Design review of the part built by this model. Coordinates are the model's own, in mm. A direction names the side the tool comes from. Coordinates: 2 decimals unless noted, no trailing zeros. Loops run counter-clockwise (first coordinate to the right, second up) from the corner with the lowest first, then second, coordinate; pieces in that order, holes last. Notation, with made-up numbers: (36.25, -27.75) - (55.25, -27.75) arc R25 ccw to (55.25, -2.75) - close; hole circle Ø7 at (29, -1). An arc over 180 degrees is marked (long way). Answer in a Markdown table with one row per item. Add a question column.
(1) For faces 4 (the face through (11.2, 1, 1.1)), 5 (the face through (9, -4.8, 15)), 6 (the face through (9.954, -11.879, 1.085)), 7 (the face through (10.301, 0, 17)), 8 (the face through (9, 4.8, 26)), list the 3-axis set-ups (+Z, -Z, +X, -X, +Y, -Y) from which the entire face can be reached by the end or side of a thin tool; tool diameter is ignored.
(2) We need section B-B, the plane z = 17. Write out the cut boundary in (x, y), plus the area to 3 significant figures.
(3) We need section D-D, the plane z = 10.25. Write out the cut boundary in (x, y).
(4) The part is to be moulded in two halves that separate along Y. For faces 1 (the face through (9, 3, 24.5)), 2 (the face through (15, 0, 0)), 3 (the face through (3, 21.056, 2)), say which applies: released by +Y, released by -Y, zero draft, split by the parting line, or undercut.
(5) We need section C-C, the plane y = 3.5. Write out the cut boundary in (x, z), plus the area to 3 significant figures.
(6) We need section A-A, the plane x = 0. Write out the cut boundary in (y, z), plus the area to 3 significant figures.
(7) Clearance check with flat-ended pins moving along their axes: pin 1 (5 mm diameter, centred on x = 0, y = 0, fed in from +Z); pin 2 (1.9 mm diameter, centred on x = 9.5, y = 3.5, fed in from +Z); pin 3 (2.5 mm diameter, centred on x = 9, z = 20.5, fed in from -Y); pin 4 (8 mm diameter, centred on x = 10.5, z = 6, fed in from -Y). State where each tip first meets the part, or that it passes through.
(8) To check wall thickness, follow L1, parallel to Y at x = 0, z = 2.9; L2, parallel to Y at x = 0, z = 4.6; L3, parallel to X at y = 0, z = 3.7. State the ranges of each line that lie inside material, in increasing order. Write a range as [from, to].
from build123d import *

# Parameters (mm, degrees)
BOSS_EXTRUDE1_DEPTH   = 2.2
BOSS_EXTRUDE1_2_DEPTH = 2.2
BOSS_EXTRUDE1_3_DEPTH = 2.2
SKETCH3_R             = 1.5
BOSS_EXTRUDE2_DEPTH   = 2.5
SKETCH4_R             = 3.05
CUT_EXTRUDE1_DEPTH    = 0.6
SKETCH5_W             = 2.4
SKETCH5_H             = 2.4
BOSS_EXTRUDE3_DEPTH   = 22.15
BOSS_EXTRUDE4_DEPTH   = 2.4
CHAMFER1_SIZE         = 2
CHAMFER1_SIZE_2       = 1.48467926


with BuildPart() as part:
    # Sketch1 → Boss-Extrude1 (new body)
    with BuildSketch(Plane.XY):
        Polygon((-3.5, 21.055685406), (-3.5, 10.2), (5.888972746, 10.2), (6.342667922, 9.414176903), (13.466375906, 14.276390289), (8.839237969, 21.055685406), align=None)
    extrude(amount=BOSS_EXTRUDE1_DEPTH)



with BuildPart() as body_2:
    # Sketch1 → Boss-Extrude1 2 (new body)
    with BuildSketch(Plane.XY):
        Polygon((18.201821848, -7.338411352), (10.554607275, -2.118883945), (11.777945491, 0), (10.554607275, 2.118883945), (18.201821848, 7.338411352), align=None)
    extrude(amount=BOSS_EXTRUDE1_2_DEPTH)


with BuildPart() as body_3:
    # Sketch1 → Boss-Extrude1 3 (new body)
    with BuildSketch(Plane.XY):
        Polygon((8.839237969, -21.055685406), (13.466375906, -14.276390289), (6.342667922, -9.414176903), (5.888972746, -10.2), (-3.5, -10.2), (-3.5, -21.055685406), align=None)
    extrude(amount=BOSS_EXTRUDE1_3_DEPTH)


with BuildPart() as part_1:
    add(part.part)

    add(body_2.part)  # Boss-Extrude2 merges body 2

    add(body_3.part)  # Boss-Extrude2 merges body 3
    # Sketch3 → Boss-Extrude2 (add)
    with BuildSketch(Plane.XY.offset(2.2)):
        Polygon((-3.5, 21.055685406), (-3.5, -21.055685406), (8.839237969, -21.055685406), (18.201821848, -7.338411352), (18.201821848, 7.338411352), (8.839237969, 21.055685406), align=None)
        Circle(SKETCH3_R, mode=Mode.SUBTRACT)
    extrude(amount=BOSS_EXTRUDE2_DEPTH)

    # Sketch4 → Cut-Extrude1 (cut)
    with BuildSketch(Plane.XY.offset(4.7)):
        Circle(SKETCH4_R)
    extrude(amount=-CUT_EXTRUDE1_DEPTH, mode=Mode.SUBTRACT)

    # Sketch5 → Boss-Extrude3 (add)
    with BuildSketch(Plane.XY.offset(4.7)):
        with Locations((9.100910924, 6)):
            Rectangle(SKETCH5_W, SKETCH5_H)
        with Locations((9.100910924, -6)):
            Rectangle(SKETCH5_W, SKETCH5_H)
    extrude(amount=BOSS_EXTRUDE3_DEPTH)

    # Sketch6 → Boss-Extrude4 (add)
    with BuildSketch(Plane(origin=(10.300910924, 0, 0), x_dir=(0, 0, -1), z_dir=(1, 0, 0))):
        Polygon((-6.387662753, 4.8), (-9.65, -1.526957086), (-12.912337247, 4.8), (-16.287662753, 4.8), (-19.55, -1.526957086), (-22.812337247, 4.8), (-24.5, 4.8), (-24.5, 1.526957086), (-21.237662753, -4.8), (-17.862337247, -4.8), (-14.6, 1.526957086), (-11.337662753, -4.8), (-7.962337247, -4.8), (-4.7, 1.526957086), (-4.7, 4.8), align=None)
    extrude(amount=-BOSS_EXTRUDE4_DEPTH)

    # Chamfer1
    # the kernel refuses this chamfer: 2, 1.48467926 mm, written as the material it adds along each edge
    with BuildSketch(Plane(origin=(15.4442769, 1.526957086, 4.7), x_dir=(0, -1, 0), z_dir=(-1, 0, 0))) as chamfer1_piece_1_section:
        Polygon((CHAMFER1_SIZE, 0), (CHAMFER1_SIZE_2 * 0.888803167403, CHAMFER1_SIZE_2 * 0.458289133192), (0, 0), align=None)
    chamfer1_piece_1 = extrude(amount=12.686731952, mode=Mode.PRIVATE)
    chamfer1_piece_1 = split(chamfer1_piece_1, bisect_by=Plane(origin=(10.672593912, 1.526957086, 9.471682988), z_dir=(0.7071067811865476, 0, -0.7071067811865476)), keep=Keep.TOP, mode=Mode.PRIVATE)
    chamfer1_piece_1 = split(chamfer1_piece_1, bisect_by=Plane(origin=(13.872593912, 1.526957086, 3.128317012), z_dir=(-0.7071067811865476, 0, -0.7071067811865476)), keep=Keep.TOP, mode=Mode.PRIVATE)
    add(chamfer1_piece_1)
    with BuildSketch(Plane(origin=(2.757544948, 7.2, 4.7), x_dir=(0, 1, 0), z_dir=(1, 0, 0))) as chamfer1_piece_2_section:
        Polygon((CHAMFER1_SIZE, 0), (0, CHAMFER1_SIZE), (0, 0), align=None)
    chamfer1_piece_2 = extrude(amount=12.686731952, mode=Mode.PRIVATE)
    chamfer1_piece_2 = split(chamfer1_piece_2, bisect_by=Plane(origin=(4.329227936, 7.2, 3.128317012), z_dir=(0.7071067811865476, 0, -0.7071067811865476)), keep=Keep.TOP, mode=Mode.PRIVATE)
    chamfer1_piece_2 = split(chamfer1_piece_2, bisect_by=Plane(origin=(7.529227936, 7.2, 9.471682988), z_dir=(-0.7071067811865476, 0, -0.7071067811865476)), keep=Keep.TOP, mode=Mode.PRIVATE)
    add(chamfer1_piece_2)
    with BuildSketch(Plane(origin=(10.300910924, 12.343365976, 4.7), x_dir=(1, 0, 0), z_dir=(0, -1, 0))) as chamfer1_piece_3_section:
        Polygon((CHAMFER1_SIZE, 0), (0, CHAMFER1_SIZE), (0, 0), align=None)
    chamfer1_piece_3 = extrude(amount=15.959774866, mode=Mode.PRIVATE)
    chamfer1_piece_3 = split(chamfer1_piece_3, bisect_by=Plane(origin=(10.300910924, 4.8, 4.7), z_dir=(0, 1, 0)), keep=Keep.TOP, mode=Mode.PRIVATE)
    chamfer1_piece_3 = split(chamfer1_piece_3, bisect_by=Plane(origin=(10.300910924, 10.771682988, 3.128317012), z_dir=(0, -0.7071067811865476, -0.7071067811865476)), keep=Keep.TOP, mode=Mode.PRIVATE)
    add(chamfer1_piece_3)
    with BuildSketch(Plane(origin=(10.300910924, 12.343365976, 4.7), x_dir=(1, 0, 0), z_dir=(0, -1, 0))) as chamfer1_piece_4_section:
        Polygon((CHAMFER1_SIZE, 0), (0, CHAMFER1_SIZE), (0, 0), align=None)
    chamfer1_piece_4 = extrude(amount=15.959774866, mode=Mode.PRIVATE)
    chamfer1_piece_4 = split(chamfer1_piece_4, bisect_by=Plane(origin=(10.300910924, 11.446474594, 2.96057429), z_dir=(0, -0.4582891331950048, -0.8888031674084939)), keep=Keep.TOP, mode=Mode.PRIVATE)
    chamfer1_piece_4 = split(chamfer1_piece_4, bisect_by=Plane(origin=(10.300910924, 5.935161531, 11.108204445), z_dir=(0, 0.7071067811865488, -0.7071067811865462)), keep=Keep.TOP, mode=Mode.PRIVATE)
    add(chamfer1_piece_4)
    with BuildSketch(Plane(origin=(10.300910924, 12.343365976, 4.7), x_dir=(1, 0, 0), z_dir=(0, -1, 0))) as chamfer1_piece_5_section:
        Polygon((CHAMFER1_SIZE, 0), (0, CHAMFER1_SIZE), (0, 0), align=None)
    chamfer1_piece_5 = extrude(amount=15.959774866, mode=Mode.PRIVATE)
    chamfer1_piece_5 = split(chamfer1_piece_5, bisect_by=Plane(origin=(10.300910924, 10.071607195, 0.294164788), z_dir=(0, 0.4582891331950048, 0.8888031674084939)), keep=Keep.TOP, mode=Mode.PRIVATE)
    chamfer1_piece_5 = split(chamfer1_piece_5, bisect_by=Plane(origin=(10.300910924, 5.935161531, 11.108204445), z_dir=(0, -0.7071067811865488, 0.7071067811865462)), keep=Keep.TOP, mode=Mode.PRIVATE)
    add(chamfer1_piece_5)
    with BuildSketch(Plane(origin=(7.900910924, -3.61640889, 4.7), x_dir=(-1, 0, 0), z_dir=(0, 1, 0))) as chamfer1_piece_6_section:
        Polygon((CHAMFER1_SIZE, 0), (0, CHAMFER1_SIZE), (0, 0), align=None)
    chamfer1_piece_6 = extrude(amount=15.959774866, mode=Mode.PRIVATE)
    chamfer1_piece_6 = split(chamfer1_piece_6, bisect_by=Plane(origin=(7.900910924, -2.53615324, 6.795041262), z_dir=(0, 0.4582891331950048, 0.8888031674084939)), keep=Keep.TOP, mode=Mode.PRIVATE)
    chamfer1_piece_6 = split(chamfer1_piece_6, bisect_by=Plane(origin=(7.900910924, -1.16128584, 9.461450764), z_dir=(0, -0.4582891331950048, -0.8888031674084939)), keep=Keep.TOP, mode=Mode.PRIVATE)
    add(chamfer1_piece_6)
    with BuildSketch(Plane(origin=(7.900910924, -3.61640889, 4.7), x_dir=(-1, 0, 0), z_dir=(0, 1, 0))) as chamfer1_piece_7_section:
        Polygon((CHAMFER1_SIZE, 0), (0, CHAMFER1_SIZE), (0, 0), align=None)
    chamfer1_piece_7 = extrude(amount=15.959774866, mode=Mode.PRIVATE)
    chamfer1_piece_7 = split(chamfer1_piece_7, bisect_by=Plane(origin=(7.900910924, -1.16128584, 9.461450764), z_dir=(0, -0.4582891331950048, -0.8888031674084939)), keep=Keep.TOP, mode=Mode.PRIVATE)
    chamfer1_piece_7 = split(chamfer1_piece_7, bisect_by=Plane(origin=(7.900910924, -2.044725902, 3.128317012), z_dir=(0, 0.7071067811865488, -0.7071067811865462)), keep=Keep.TOP, mode=Mode.PRIVATE)
    add(chamfer1_piece_7)
    with BuildSketch(Plane(origin=(7.900910924, -3.61640889, 4.7), x_dir=(-1, 0, 0), z_dir=(0, 1, 0))) as chamfer1_piece_8_section:
        Polygon((CHAMFER1_SIZE, 0), (0, CHAMFER1_SIZE), (0, 0), align=None)
    chamfer1_piece_8 = extrude(amount=15.959774866, mode=Mode.PRIVATE)
    chamfer1_piece_8 = split(chamfer1_piece_8, bisect_by=Plane(origin=(7.900910924, 4.8, 4.7), z_dir=(0, 1, 0)), keep=Keep.TOP, mode=Mode.PRIVATE)
    chamfer1_piece_8 = split(chamfer1_piece_8, bisect_by=Plane(origin=(7.900910924, 2.791795555, 11.108204445), z_dir=(0, -0.7071067811865476, -0.7071067811865476)), keep=Keep.TOP, mode=Mode.PRIVATE)
    add(chamfer1_piece_8)
    with BuildSketch(Plane(origin=(2.757544948, -4.8, 4.7), x_dir=(0, 1, 0), z_dir=(1, 0, 0))) as chamfer1_piece_9_section:
        Polygon((CHAMFER1_SIZE, 0), (0, CHAMFER1_SIZE), (0, 0), align=None)
    chamfer1_piece_9 = extrude(amount=12.686731952, mode=Mode.PRIVATE)
    chamfer1_piece_9 = split(chamfer1_piece_9, bisect_by=Plane(origin=(4.329227936, -4.8, 3.128317012), z_dir=(0.7071067811865476, 0, -0.7071067811865476)), keep=Keep.TOP, mode=Mode.PRIVATE)
    chamfer1_piece_9 = split(chamfer1_piece_9, bisect_by=Plane(origin=(7.529227936, -4.8, 9.471682988), z_dir=(-0.7071067811865476, 0, -0.7071067811865476)), keep=Keep.TOP, mode=Mode.PRIVATE)
    add(chamfer1_piece_9)
    with BuildSketch(Plane(origin=(10.300910924, 0.343365976, 4.7), x_dir=(1, 0, 0), z_dir=(0, -1, 0))) as chamfer1_piece_10_section:
        Polygon((CHAMFER1_SIZE, 0), (0, CHAMFER1_SIZE), (0, 0), align=None)
    chamfer1_piece_10 = extrude(amount=12.686731952, mode=Mode.PRIVATE)
    chamfer1_piece_10 = split(chamfer1_piece_10, bisect_by=Plane(origin=(10.300910924, 0.59195435, 5.182110786), z_dir=(0, 0.4582891331950048, 0.8888031674084939)), keep=Keep.TOP, mode=Mode.PRIVATE)
    add(chamfer1_piece_10)
    with BuildSketch(Plane(origin=(10.300910924, 0.343365976, 4.7), x_dir=(1, 0, 0), z_dir=(0, -1, 0))) as chamfer1_piece_11_section:
        Polygon((CHAMFER1_SIZE, 0), (0, CHAMFER1_SIZE), (0, 0), align=None)
    chamfer1_piece_11 = extrude(amount=12.686731952, mode=Mode.PRIVATE)
    chamfer1_piece_11 = split(chamfer1_piece_11, bisect_by=Plane(origin=(10.300910924, -4.428317012, 9.471682988), z_dir=(0, 0.7071067811865477, -0.7071067811865474)), keep=Keep.TOP, mode=Mode.PRIVATE)
    chamfer1_piece_11 = split(chamfer1_piece_11, bisect_by=Plane(origin=(10.300910924, -1.228317012, 3.128317012), z_dir=(0, -0.7071067811865476, -0.7071067811865476)), keep=Keep.TOP, mode=Mode.PRIVATE)
    add(chamfer1_piece_11)
    with BuildSketch(Plane(origin=(15.4442769, -7.2, 4.7), x_dir=(0, -1, 0), z_dir=(-1, 0, 0))) as chamfer1_piece_12_section:
        Polygon((CHAMFER1_SIZE, 0), (0, CHAMFER1_SIZE), (0, 0), align=None)
    chamfer1_piece_12 = extrude(amount=12.686731952, mode=Mode.PRIVATE)
    chamfer1_piece_12 = split(chamfer1_piece_12, bisect_by=Plane(origin=(10.672593912, -7.2, 9.471682988), z_dir=(0.7071067811865476, 0, -0.7071067811865476)), keep=Keep.TOP, mode=Mode.PRIVATE)
    chamfer1_piece_12 = split(chamfer1_piece_12, bisect_by=Plane(origin=(13.872593912, -7.2, 3.128317012), z_dir=(-0.7071067811865476, 0, -0.7071067811865476)), keep=Keep.TOP, mode=Mode.PRIVATE)
    add(chamfer1_piece_12)
    with BuildSketch(Plane(origin=(7.900910924, -12.343365976, 4.7), x_dir=(-1, 0, 0), z_dir=(0, 1, 0))) as chamfer1_piece_13_section:
        Polygon((CHAMFER1_SIZE, 0), (0, CHAMFER1_SIZE), (0, 0), align=None)
    chamfer1_piece_13 = extrude(amount=12.686731952, mode=Mode.PRIVATE)
    chamfer1_piece_13 = split(chamfer1_piece_13, bisect_by=Plane(origin=(7.900910924, -10.771682988, 3.128317012), z_dir=(0, 0.7071067811865477, -0.7071067811865474)), keep=Keep.TOP, mode=Mode.PRIVATE)
    chamfer1_piece_13 = split(chamfer1_piece_13, bisect_by=Plane(origin=(7.900910924, -7.571682988, 9.471682988), z_dir=(0, -0.7071067811865476, -0.7071067811865476)), keep=Keep.TOP, mode=Mode.PRIVATE)
    add(chamfer1_piece_13)
    with BuildSketch(Plane(origin=(7.900910924, -12.343365976, 4.7), x_dir=(-1, 0, 0), z_dir=(0, 1, 0))) as chamfer1_piece_14_section:
        Polygon((CHAMFER1_SIZE, 0), (0, CHAMFER1_SIZE), (0, 0), align=None)
    chamfer1_piece_14 = extrude(amount=12.686731952, mode=Mode.PRIVATE)
    chamfer1_piece_14 = split(chamfer1_piece_14, bisect_by=Plane(origin=(7.900910924, -9.43019687, 10.349782509), z_dir=(0, 0.4582891331950048, 0.8888031674084939)), keep=Keep.TOP, mode=Mode.PRIVATE)
    add(chamfer1_piece_14)


solid = part_1.part
Responses:
| question | item | result |
|---|---|---|
| 1 | face 4 | -Z, -X |
| 1 | face 5 | +X, -X |
| 1 | face 6 | -Z, +X |
| 1 | face 7 | +Z, +X, +Y, -Y |
| 1 | face 8 | +Z, +X, -X |
| 2 | outline | (7.9, -7.2) - (10.3, -7.2) - (10.3, -4.8) - (7.9, -4.8) - close; (7.9, -3.13) - (10.3, -3.13) - (10.3, 3.42) - (7.9, 3.42) - close; (7.9, 4.8) - (10.3, 4.8) - (10.3, 7.2) - (7.9, 7.2) - close |
| 2 | area | 27.2 mm2 |
| 3 | outline | (7.9, -7.2) - (10.3, -7.2) - (10.3, -0.36) - (7.9, -0.36) - close; (7.9, 4.8) - (10.3, 4.8) - (10.3, 7.2) - (7.9, 7.2) - close |
| 4 | face 1 | undercut |
| 4 | face 2 | zero draft |
| 4 | face 3 | released by +Y |
| 5 | outline | (-3.5, 2.2) - (12.58, 2.2) - (12.58, 0) - (18.2, 0) - (18.2, 4.7) - (12.3, 4.7) - (10.3, 6.7) - (10.3, 7.06) - (7.9, 7.06) - (7.9, 6.7) - (5.9, 4.7) - (-3.5, 4.7) - close; (7.9, 12.24) - (10.3, 12.24) - (10.3, 16.96) - (7.9, 16.96) - close; (7.9, 22.14) - (10.3, 22.14) - (10.3, 24.5) - (7.9, 24.5) - close |
| 5 | area | 93.3 mm2 |
| 6 | outline | (-21.06, 0) - (-10.2, 0) - (-10.2, 2.2) - (-1.5, 2.2) - (-1.5, 4.1) - (-3.05, 4.1) - (-3.05, 4.7) - (-21.06, 4.7) - close; (1.5, 2.2) - (10.2, 2.2) - (10.2, 0) - (21.06, 0) - (21.06, 4.7) - (3.05, 4.7) - (3.05, 4.1) - (1.5, 4.1) - close |
| 6 | area | 144 mm2 |
| 7 | pin 1 | stops at z = 4.1 |
| 7 | pin 2 | stops at z = 24.5 |
| 7 | pin 3 | stops at y = -7.2 |
| 7 | pin 4 | stops at y = -21.06 |
| 8 | L1 | y = [-21.06, -1.5], [1.5, 21.06] |
| 8 | L2 | y = [-21.06, -3.05], [3.05, 21.06] |
| 8 | L3 | x = [-3.5, -1.5], [1.5, 18.2] |
